The model under review builds one solid part; all positions refer to its coordinate system, in mm. Round coordinates to 2 decimals unless told otherwise and drop trailing zeros. Write each loop counter-clockwise with the first axis right and the second up, starting at its lowest first coordinate (ties: lowest second). Pieces come first, ordered by that corner, then holes. Notation, with made-up numbers: M 40,27 L 98,27 A11 cw 98,42 Z; hole C -14.5,-39.75 d3. An arc over 180 degrees is marked long. Write item = value, one per line. Start each with the question number.
Item 1: Take a section at B-B, the plane z = -2.05. Give the boundary of the cut face in (x, y), plus the area to 3 significant figures.
Item 2: To check wall thickness, follow line 1 along Y through (x, z) = (10.5, -1.7). State the ranges of the line that lie inside material, in increasing order.
Item 3: Take a section at C-C, the plane y = 2.5. Give the boundary of the cut face in (x, z).
Item 4: Take a section at A-A, the plane x = -10.5. Give the boundary of the cut face in (y, z), plus the area to 3 significant figures.
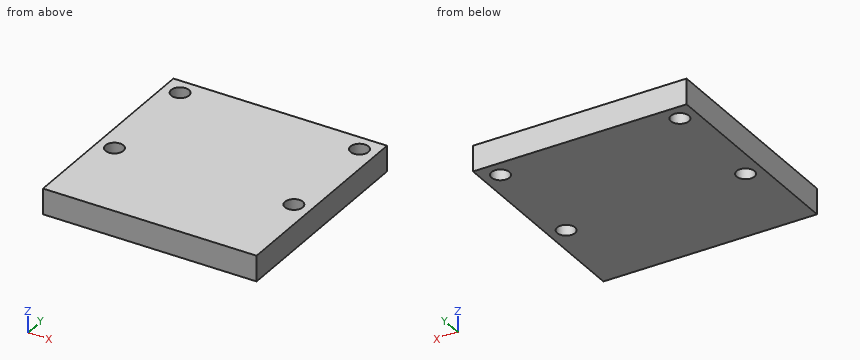
Autodesk Inventor part; units mm, degrees
ref_plane "Plano de trabajo1" through (10.95, 6.5, 0) normal (0, 0, -1) x (-1, 0, 0)
ref_plane "YZ Plane" through (0, 0, 0) normal (1, 0, 0) x (0, 1, 0)
ref_plane "XZ Plane" through (0, 0, 0) normal (0, 1, 0) x (-1, 0, 0)
ref_plane "Plano de trabajo1" through (10.95, 6.5, 0) normal (0, 0, -1) x (-1, 0, 0)
sketch "Boceto1" plane through (10.95, 6.5, 0) normal (0, 0, -1) x (-1, 0, 0)
  circle A0 centre (0.45, -4) radius 1.05
  circle A1 centre (21.45, -4) radius 1.05
  circle A2 centre (21.45, -16.58) radius 1.05
  circle A3 centre (0.45, -16.58) radius 1.05
  line L0 (-1.55, 3.5) -> (-1.55, -16.5)
  line L1 (0.45, -18.5) -> (21.45, -18.5)
  line L2 (23.45, -16.5) -> (23.45, 3.5)
  line L3 (-1.55, -2) -> (23.45, -2)
  line L4 (23.45, -2) -> (23.45, -27)
  line L5 (23.45, -27) -> (-1.55, -27)
  line L6 (-1.55, -27) -> (-1.55, -2)
  circle A4 centre (0.45, -4) radius 1.05
  circle A5 centre (21.45, -4) radius 1.05
  circle A6 centre (0.45, -16.58) radius 1.05
  circle A7 centre (21.45, -16.58) radius 1.05
  point P0 (10.95, -6.5)
  point P1 (0, 0)
  dimension "d1" = 2
  dimension "d3" = 25
extrude "Extrusión1" add sketch "Boceto1" along normal blind 3
properties part number "RPi_Camera_V2.1"
Response values:
q1.outline = M -12.5,-20.5 L 12.5,-20.5 L 12.5,4.5 L -12.5,4.5 Z; hole C -10.5,-10.08 d2.1; hole C -10.5,2.5 d2.1; hole C 10.5,-10.08 d2.1; hole C 10.5,2.5 d2.1
q1.area = 611 mm2
q2.line_1 = -20.5 to -11.13, -9.03 to 1.45, 3.55 to 4.5
q3.outline = M -12.5,-3 L -11.55,-3 L -11.55,0 L -12.5,0 Z; M -9.45,-3 L 9.45,-3 L 9.45,0 L -9.45,0 Z; M 11.55,-3 L 12.5,-3 L 12.5,0 L 11.55,0 Z
q4.outline = M -20.5,-3 L -11.13,-3 L -11.13,0 L -20.5,0 Z; M -9.03,-3 L 1.45,-3 L 1.45,0 L -9.03,0 Z; M 3.55,-3 L 4.5,-3 L 4.5,0 L 3.55,0 Z
q4.area = 62.4 mm2
